Here's how the part is built. I have some questions about the finished solid (model axes, mm). Round coordinates to 2 decimals unless told otherwise and drop trailing zeros. Write each loop counter-clockwise with the first axis right and the second up, starting at its lowest first coordinate (ties: lowest second). Pieces come first, ordered by that corner, then holes. Notation, with made-up numbers: (-16.5, 54.5) - (12.5, 54.5) arc R18 cw to (12.5, 75.5) - close; hole circle Ø3 at (55.5, 12.25). An arc over 180 degrees is marked (long way). Return JSON: item names as keys, results as strings. Group by question number.
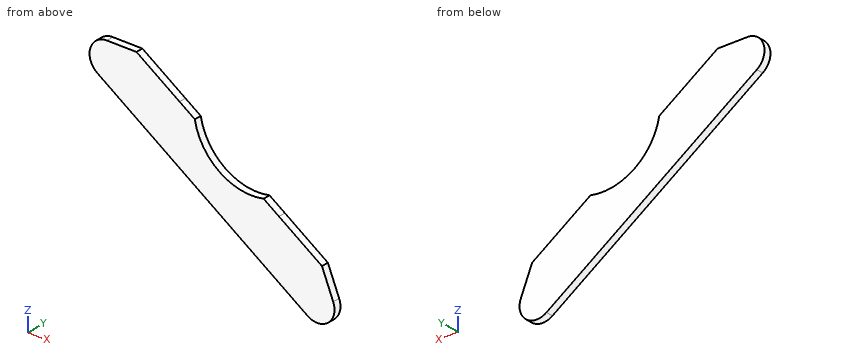
Autodesk Inventor part; units mm, degrees
ref_plane "YZ Plane" through (0, 0, 0) normal (1, 0, 0) x (0, 1, 0)
ref_plane "XZ Plane" through (0, 0, 0) normal (0, 1, 0) x (-1, 0, 0)
ref_plane "XY Plane" through (0, 0, 0) normal (0, 0, 1) x (1, 0, 0)
sketch "Sketch1" plane through (0, 0, 0) normal (0, 1, 0) x (-1, 0, 0)
  circle A0 centre (0, 0) radius 19.812
  line L0 (69.85, 0) -> (31.75, 0)
  line L1 (-12.0631, -29.3691) -> (-26.5388, -64.612)
  line L2 (-26.5388, -64.612) -> (69.85, 0)
  line L3 (69.85, 0) -> (88.796, 12.7)
  line L4 (88.796, 12.7) -> (50.696, 12.7)
  line L5 (50.696, 12.7) -> (31.75, 0)
  line L6 (-12.0631, -29.3691) -> (-31.0091, -42.0691)
  line L7 (-31.0091, -42.0691) -> (-45.4848, -77.312)
  line L8 (-45.4848, -77.312) -> (-26.5388, -64.612)
  arc A1 (-5.306, -24.8396) -> (24.9929, -4.5295) centre (0, 0) ccw
  line L9 (31.75, 0) -> (24.9929, -4.5295)
  line L10 (-5.306, -24.8396) -> (-12.0631, -29.3691)
  dimension "d0" = 112.33
  dimension "d2" = 39.624
  dimension "d3" = 31.75
  dimension "d4" = 31.75
  dimension "d5" = 38.1
  dimension "d6" = 38.1
  dimension "d7" = 112.33
  dimension "d10" = 12.7
  dimension "d12" = 12.7
  dimension "d13" = 25.4
extrude "Extrusion1" add sketch "Sketch1" along normal blind 3.175 contours L2 L1 L10 A1 L9 L0 | L0 L5 L4 L3 | L8 L7 L6 L1
sketch "Sketch2" plane through (0, 0, 0) normal (0, -1, 0) x (1, 0, 0)
  line L0 (45.4848, -77.312) -> (-88.796, 12.7)
  line L1 (31.0091, -42.0691) -> (45.4848, -77.312)
  line L2 (5.306, -24.8396) -> (31.0091, -42.0691)
  arc A0 (-24.9929, -4.5295) -> (5.306, -24.8396) centre (0, 0) ccw
  line L3 (-50.696, 12.7) -> (-24.9929, -4.5295)
  line L4 (-88.796, 12.7) -> (-50.696, 12.7)
fillet "Fillet1" radius 7.62 2 edges at (-88.796, 1.5875, 12.7) (45.4848, 1.5875, -77.312)
properties part number "gusset" material "Stainless Steel"
1) Imagine slicing it at A-A (z = -33.5). Please give me the cut outline in (x, y) (3 decimals), plus the area to 3 significant figures.
2) I need wall thicknesses on line 1 along X through (y, z) = (2.15, -36); line 2 along Z through (x, y) = (-5, 0.2); line 3 along X through (y, z) = (1.65, 2). Which ranges of each line are inside material? Lowest first, please.
3) Imagine slicing it at B-B (x = 22). Please give me the cut outline in (y, z) (3 decimals).
4) Will these pins go through, and if not, where does the flat tip stop? pin 1 Ø10 at (x, z) = (-11.5, -40) entering from +Y (3 decimals); pin 2 Ø10 at (x, z) = (24.5, -31.5) entering from +Y; pin 3 Ø1.5 at (y, z) = (2, -21.5) entering from -X.
Results found:
{
 "1": {"outline": "(-19.874, 0) - (18.226, 0) - (18.226, 3.175) - (-19.874, 3.175) - close", "area": "121 mm²"},
 "2": {"line 1": "x = -16.14 to 21.96", "line 2": "z = -43.47 to -24.9", "line 3": "x = -70.71 to -34.73"},
 "3": {"outline": "(0, -61.57) - (3.175, -61.57) - (3.175, -36.03) - (0, -36.03) - close"},
 "4": {"pin 1": "stops at y = 3.175", "pin 2": "passes through", "pin 3": "stops at x = -38.89"}
}
